from build123d import *

# Parameters (mm, degrees)
BOSS_EXTRUDE1_DEPTH = 21
SKETCH2_R           = 5.34
CUT_EXTRUDE1_DEPTH  = 7
CUT_EXTRUDE2_DEPTH  = 39.078996836
CHAMFER1_SIZE       = 0.4
FILLET1_R           = 10
SKETCH4_R           = 1
CUT_EXTRUDE3_DEPTH  = 8.125
SKETCH6_R           = 4.15
BOSS_EXTRUDE2_DEPTH = 21
FILLET2_R           = 10
SKETCH5_R           = 1.5
CUT_EXTRUDE5_DEPTH  = 4.2
SKETCH7_R           = 3.025
CUT_EXTRUDE6_DEPTH  = 9
FILLET3_R           = 0.2
SKETCH8_W           = 0.96
SKETCH8_H           = 4
BOSS_EXTRUDE3_DEPTH = 21
FILLET4_R           = 1
SKETCH10_R          = 1.7
CUT_EXTRUDE7_DEPTH  = 43.006695945
SKETCH12_W          = 4
SKETCH12_H          = 1
CUT_EXTRUDE8_DEPTH  = 42.542899564


with BuildPart() as part:
    # Sketch1 → Boss-Extrude1 (new body)
    with BuildSketch(Plane.XY):
        with BuildLine():
            Line((-23.445643943, -2.5), (31.1, -2.5))
            ThreePointArc((31.1, -2.5), (33.6, 0), (31.1, 2.5))
            Line((31.1, 2.5), (-23.445643943, 2.5))
            ThreePointArc((-23.445643943, 2.5), (-34.9, 0), (-23.445643943, -2.5))
        make_face()
    extrude(amount=BOSS_EXTRUDE1_DEPTH)

    # Sketch2 → Cut-Extrude1 (cut)
    with BuildSketch(Plane.XY.offset(21)):
        with Locations((-28.9, 0)):
            Circle(SKETCH2_R)
    extrude(amount=-CUT_EXTRUDE1_DEPTH, mode=Mode.SUBTRACT)

    # Sketch3 → Cut-Extrude2 (cut, through all)
    with BuildSketch(Plane.XY.offset(14)):
        with BuildLine():
            Line((-33.19, 3.179858487), (-33.19, -3.179858487))
            ThreePointArc((-33.19, -3.179858487), (-28.9, -5.34), (-24.61, -3.179858487))
            Line((-24.61, -3.179858487), (-24.61, 3.179858487))
            ThreePointArc((-24.61, 3.179858487), (-28.9, 5.34), (-33.19, 3.179858487))
        make_face()
    extrude(amount=-CUT_EXTRUDE2_DEPTH, mode=Mode.SUBTRACT)

    # Chamfer1
    # the kernel refuses this chamfer: 0.4 mm, written as the material it takes off along each edge
    with BuildSketch(Plane(origin=(-24.61, -4.208531683, 14), x_dir=(-0.027495876610587302, 0, -0.9996219169112966), z_dir=(0, 1, 0))) as chamfer1_piece_1_section:
        Polygon((CHAMFER1_SIZE * 0.999621916911, -CHAMFER1_SIZE * 0.0274958766106), (-CHAMFER1_SIZE * 0.0274958766106, -CHAMFER1_SIZE * 0.999621916911), (0, 0), align=None)
    chamfer1_piece_1 = extrude(amount=8.417063365, mode=Mode.PRIVATE)
    chamfer1_piece_1 = chamfer1_piece_1 & Plane(origin=(-28.9, 0, 13.865333272), x_dir=(0.803370786516886, 0.595479117493838, 0), z_dir=(0, 0, 1)) * Cylinder(5.34, 19, mode=Mode.PRIVATE)
    add(chamfer1_piece_1, mode=Mode.SUBTRACT)
    with BuildSketch(Plane(origin=(-33.19, 4.208531683, 14), x_dir=(0.027495876610578673, 0, -0.999621916911297), z_dir=(0, -1, 0))) as chamfer1_piece_2_section:
        Polygon((CHAMFER1_SIZE * 0.999621916911, -CHAMFER1_SIZE * 0.0274958766106), (-CHAMFER1_SIZE * 0.0274958766106, -CHAMFER1_SIZE * 0.999621916911), (0, 0), align=None)
    chamfer1_piece_2 = extrude(amount=8.417063365, mode=Mode.PRIVATE)
    chamfer1_piece_2 = chamfer1_piece_2 & Plane(origin=(-28.9, 0, 13.865333272), x_dir=(0.803370786516886, 0.595479117493838, 0), z_dir=(0, 0, 1)) * Cylinder(5.34, 19, mode=Mode.PRIVATE)
    add(chamfer1_piece_2, mode=Mode.SUBTRACT)

    # Fillet1
    fillet1_edges = [part.edges().sort_by_distance(p)[0] for p in [
        (-23.445643943, 2.5, 10.5),
        (-23.445643943, -2.5, 10.5),
    ]]
    fillet(fillet1_edges, radius=FILLET1_R)

    # Sketch4 → Cut-Extrude3 (cut, symmetric)
    with BuildSketch(Plane(origin=(0, 0, 0), x_dir=(1, 0, 0), z_dir=(0, 1, 0))):
        with Locations((-30.027345217, -3)):
            Circle(SKETCH4_R)
        with BuildLine():
            ThreePointArc((-31.027345217, -3), (-30.027345217, -2), (-29.027345217, -3))
            Line((-29.027345217, -3), (-29.027345217, 4))
            Line((-29.027345217, 4), (-31.027345217, 4))
            Line((-31.027345217, 4), (-31.027345217, -3))
        make_face()
    extrude(amount=CUT_EXTRUDE3_DEPTH, both=True, mode=Mode.SUBTRACT)

    # Sketch6 → Boss-Extrude2 (add, through all)
    with BuildSketch(Plane.XY.offset(21)):
        with Locations((31.1, 0)):
            Circle(SKETCH6_R)
    extrude(amount=-BOSS_EXTRUDE2_DEPTH)

    # Fillet2
    fillet2_edges = [part.edges().sort_by_distance(p)[0] for p in [
        (27.787523585, 2.5, 10.5),
        (27.787523585, -2.5, 10.5),
    ]]
    fillet(fillet2_edges, radius=FILLET2_R)

    # Sketch5 → Cut-Extrude5 (cut)
    with BuildSketch(Plane(origin=(0, 0, 0), x_dir=(-1, 0, 0), z_dir=(0, 0, -1))):
        with Locations((-31.1, 0)):
            Circle(SKETCH5_R)
        with Locations((-6.1, 0)):
            Circle(SKETCH5_R)
        with Locations((18.9, 0)):
            Circle(SKETCH5_R)
    extrude(amount=-CUT_EXTRUDE5_DEPTH, mode=Mode.SUBTRACT)

    # Sketch7 → Cut-Extrude6 (cut)
    with BuildSketch(Plane.XY.offset(21)):
        with Locations((31.1, 0)):
            Circle(SKETCH7_R)
    extrude(amount=-CUT_EXTRUDE6_DEPTH, mode=Mode.SUBTRACT)

    # Fillet3
    fillet3_edges = [part.edges().sort_by_distance(p)[0] for p in [
        (28.075, 0, 21),
        (-34.24, 0, 21),
    ]]
    fillet(fillet3_edges, radius=FILLET3_R)

    # Sketch8 → Boss-Extrude3 (add, through all)
    with BuildSketch(Plane.XY.offset(21)):
        with Locations((21.258157906, 4.5)):
            Rectangle(SKETCH8_W, SKETCH8_H)
        with Locations((24.298157906, 4.5)):
            Rectangle(SKETCH8_W, SKETCH8_H)
        with Locations((21.258157906, -4.5)):
            Rectangle(SKETCH8_W, SKETCH8_H)
        with Locations((24.298157906, -4.5)):
            Rectangle(SKETCH8_W, SKETCH8_H)
    extrude(amount=-BOSS_EXTRUDE3_DEPTH)

    # Fillet4
    fillet4_edges = [part.edges().sort_by_distance(p)[0] for p in [
        (20.778157906, 2.5, 10.5),
        (24.778157906, 2.50478553, 10.5),
        (20.778157906, -2.5, 10.5),
        (24.778157906, -2.50478553, 10.5),
    ]]
    fillet(fillet4_edges, radius=FILLET4_R)

    # Sketch10 → Cut-Extrude7 (cut, through all)
    with BuildSketch(Plane(origin=(0, 2.5, 0), x_dir=(1, 0, 0), z_dir=(0, 1, 0))):
        with Locations(Location((-14.648773097, -17, 0), (0, 0, 180))):
            Circle(SKETCH10_R)
        with Locations(Location((0.351226903, -17, 0), (0, 0, 180))):
            Circle(SKETCH10_R)
        with Locations(Location((15.351226903, -17, 0), (0, 0, 180))):
            Circle(SKETCH10_R)
        with Locations(Location((0.351226903, -3, 0), (0, 0, 180))):
            Circle(SKETCH10_R)
        with Locations(Location((15.351226903, -3, 0), (0, 0, 180))):
            Circle(SKETCH10_R)
        with Locations(Location((-14.648773097, -3, 0), (0, 0, 180))):
            Circle(SKETCH10_R)
    extrude(amount=-CUT_EXTRUDE7_DEPTH, mode=Mode.SUBTRACT)

    # Sketch12 → Cut-Extrude8 (cut, through all)
    with BuildSketch(Plane.XY.offset(21)):
        with Locations((22.778157906, 6)):
            Rectangle(SKETCH12_W, SKETCH12_H)
        with Locations((22.778157906, -6)):
            Rectangle(SKETCH12_W, SKETCH12_H)
    extrude(amount=-CUT_EXTRUDE8_DEPTH, mode=Mode.SUBTRACT)


solid = part.part
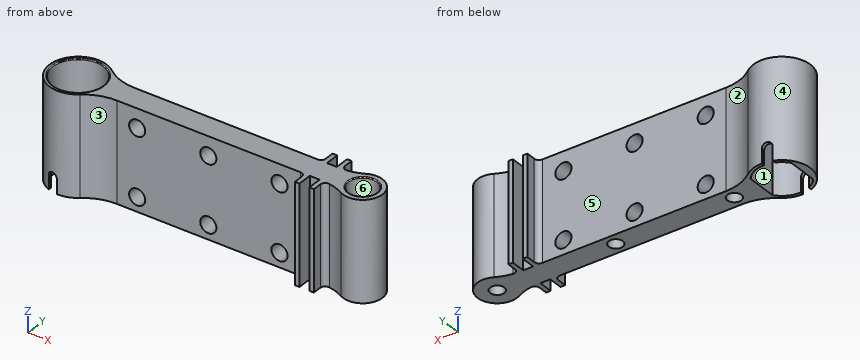
The model under review builds one solid part; all positions refer to its coordinate system, in mm. Face numbers are marked on the shaded views. A direction names the side the tool comes from. Round coordinates to 2 decimals unless told otherwise and drop trailing zeros. Loops run counter-clockwise (first coordinate to the right, second up) from the corner with the lowest first, then second, coordinate; pieces in that order, holes last. Notation, with made-up numbers: M 37,-4 L 58,-4 A11 ccw 58,14 Z; hole C 70,74 d8. An arc over 180 degrees is marked long. Answer as CSV lines item,"result".
1. Insertion check: pin 1 Ø5.5 at (x, z) = (0.35, 3) entering from +Y; pin 2 Ø5.5 at (x, z) = (0.35, 17) entering from -Y; pin 3 Ø2 at (x, z) = (15.35, 17) entering from +Y; pin 4 Ø0.9 at (y, z) = (-4, 11.5) entering from +X. Each pin has a flat end and moves straight along its axis. Give the tip position at first contact, or say it passes through.
Outcome:
pin 1,"stops at y = 2.5"
pin 2,"stops at y = -2.5"
pin 3,"passes through"
pin 4,"stops at x = 33.25"
2. To check wall thickness, follow L1, parallel to Y at x = 6.1, z = 1.5; L2, parallel to X at y = 0, z = 7.75; L3, parallel to X at y = 3.75, z = 10.75. State the ranges of each line that lie inside material, in increasing order. Write a range as [from, to].
Outcome:
L1,"y = [-2.5, -1.5], [1.5, 2.5]"
L2,"x = [-34.9, -33.19], [-24.61, 35.25]"
L3,"x = [-33.58, -32.7], [-25.1, -23.75], [20.78, 21.74], [23.82, 24.78], [29.32, 32.88]"
3. For the marked faces 1, 2 and 3, list the 3-axis set-ups (+Z, -Z, +X, -X, +Y, -Y) from which the entire face can be reached by the end or side of a thin tool; tool diameter is ignored.
Outcome:
face 1,"+Z, -Z"
face 2,"+Z, -Z, +Y"
face 3,"+Z, -Z, -Y"
4. We need section C-C (x = 31.1). Give the boundary of the cut face in (y, z) (3 decimals).
Outcome:
outline,"M -4.15,0 L -1.5,0 L -1.5,4.2 L 1.5,4.2 L 1.5,0 L 4.15,0 L 4.15,21 L 3.225,21 A0.2 ccw 3.025,20.8 L 3.025,12 L -3.025,12 L -3.025,20.8 A0.2 ccw -3.225,21 L -4.15,21 Z"
5. Draft analysis for pull direction Y (two halves, no side actions). For the marked faces 4, 5 and 6, state which applies: pulls with the +Y half, pulls with the -Y half, needs draft (parallel to the pull), parting line crosses it, or undercut.
Outcome:
face 4,"parting line crosses it"
face 5,"pulls with the +Y half"
face 6,"undercut"
6. We need section D-D (x = 6.1). Give the boundary of the cut face in (y, z), plus the area to 3 significant figures.
Outcome:
outline,"M -2.5,0 L -1.5,0 L -1.5,4.2 L 1.5,4.2 L 1.5,0 L 2.5,0 L 2.5,21 L -2.5,21 Z"
area,"92.4 mm2"
7. We need section A-A (y = 0). Count the separate pieces of the cut face and the enclosed holes in it, plus the area to 3 significant figures.
Outcome:
separate pieces,"2"
enclosed holes,"6"
area,"1,130 mm2"
